```python
from build123d import *

# Parameters (mm, degrees)
SKETCH1_R                = 8.5
BOSS_EXTRUDE1_DEPTH      = 2
BOSS_EXTRUDE2_DEPTH      = 4
BOSS_EXTRUDE2_DEPTH_BACK = 2
CHAMFER1_SIZE            = 1
CHAMFER1_SIZE2           = 2.050303842
CUT_EXTRUDE1_DEPTH       = 1
SKETCH5_W                = 5
SKETCH5_H                = 2.5
BOSS_EXTRUDE3_DEPTH      = 6
CHAMFER2_SIZE            = 3.8


with BuildPart() as part:
    # Sketch1 → Boss-Extrude1 (new body)
    # profile 1 of 2: a face of its own
    with BuildSketch(Plane.XY):
        with BuildLine():
            Line((-22.564385508, -10.000007952), (-6, -10.000007952))
            Line((-6, -10.000007952), (-6, -7.5))
            ThreePointArc((-6, -7.5), (-5.267766953, -5.732233047), (-3.5, -5))
            Line((-3.5, -5), (3.5, -5))
            ThreePointArc((3.5, -5), (5.267766953, -5.732233047), (6, -7.5))
            Line((6, -7.5), (6, -10.000007952))
            Line((6, -10.000007952), (22.435614492, -10.000007952))
            Line((22.435614492, -10.000007952), (22.435614492, 9.999992048))
            Line((22.435614492, 9.999992048), (-22.564385508, 9.999992048))
            Line((-22.564385508, 9.999992048), (-22.564385508, -10.000007952))
        make_face()
        with Locations((-13, 0)):
            Circle(SKETCH1_R, mode=Mode.SUBTRACT)
        with Locations((13, 0)):
            Circle(SKETCH1_R, mode=Mode.SUBTRACT)
    # profile 2 of 2: a face of its own
    with BuildSketch(Plane.XY):
        Polygon((-6, -10.500007952), (-6, -10.000007952), (-22.564385508, -10.000007952), (-22.564385508, 9.999992048), (22.435614492, 9.999992048), (22.435614492, -10.000007952), (6, -10.000007952), (6, -10.500007952), (22.935614492, -10.500007952), (22.935614492, 10.499992048), (-23.064385508, 10.499992048), (-23.064385508, -10.500007952), align=None)
    extrude(amount=BOSS_EXTRUDE1_DEPTH)

    # Sketch2 → Boss-Extrude2 (add, two sides: drawn at the far end of the back side and taken through both)
    with BuildSketch(Plane(origin=(0, 0, 0), x_dir=(-1, 0, 0), z_dir=(0, 0, -1)).offset(-BOSS_EXTRUDE2_DEPTH_BACK)):
        Polygon((6, -12.500007952), (25.064385508, -12.500007952), (25.064385508, 12.499992048), (-24.935614492, 12.499992048), (-24.935614492, -12.500007952), (-6, -12.500007952), (-6, -10.500007952), (-22.935614492, -10.500007952), (-22.935614492, 10.499992048), (23.064385508, 10.499992048), (23.064385508, -10.500007952), (6, -10.500007952), align=None)
    extrude(amount=BOSS_EXTRUDE2_DEPTH + BOSS_EXTRUDE2_DEPTH_BACK)

    # Chamfer1
    chamfer1_edges = [part.edges().sort_by_distance(p)[0] for p in [
        (-15.532192754, -12.500007952, 2),
        (-25.064385508, -7.952e-06, 2),
        (-0.064385508, 12.499992048, 2),
        (24.935614492, -7.952e-06, 2),
        (15.467807246, -12.500007952, 2),
    ]]
    chamfer1_side = [part.faces().sort_by_distance(p)[0] for p in [
        (-0.113559128, 1.090103523, 2),
    ]]
    chamfer(chamfer1_edges, length=CHAMFER1_SIZE, length2=CHAMFER1_SIZE2, reference=chamfer1_side[0])

    # Sketch3 → Cut-Extrude1 (cut)
    with BuildSketch(Plane(origin=(0, 0, 0), x_dir=(-1, 0, 0), z_dir=(0, 0, -1))):
        with BuildLine():
            Line((-5, 9.949992048), (5, 9.949992048))
            ThreePointArc((5, 9.949992048), (6.2, 8.749992048), (5, 7.549992048))
            Line((5, 7.549992048), (-5, 7.549992048))
            ThreePointArc((-5, 7.549992048), (-6.2, 8.749992048), (-5, 9.949992048))
        make_face()
    extrude(amount=-CUT_EXTRUDE1_DEPTH, mode=Mode.SUBTRACT)

    # Sketch5 → Boss-Extrude3 (add)
    with BuildSketch(Plane.XZ.offset(-10.499992048)):
        with Locations((7.5, -5.25)):
            Rectangle(SKETCH5_W, SKETCH5_H)
        Polygon((10, -6.5), (5, -6.5), (5, -9), (12.5, -9), (12.5, -6.5), align=None)
        with Locations((-7.5, -5.25)):
            Rectangle(SKETCH5_W, SKETCH5_H)
        Polygon((-5, -9), (-5, -6.5), (-10, -6.5), (-12.5, -6.5), (-12.5, -9), align=None)
    extrude(amount=-BOSS_EXTRUDE3_DEPTH)

    # Chamfer2
    chamfer2_edges = [part.edges().sort_by_distance(p)[0] for p in [
        (7.5, 12.499992048, -4),
        (-7.5, 12.499992048, -4),
    ]]
    chamfer(chamfer2_edges, length=CHAMFER2_SIZE)


solid = part.part
```
Model file for the job. Use its own axes, mm. A direction names the side the tool comes from. Coordinates: 2 decimals unless noted, no trailing zeros. Loops run counter-clockwise (first coordinate to the right, second up) from the corner with the lowest first, then second, coordinate; pieces in that order, holes last. Notation, with made-up numbers: M 7.5,62 L 14.5,62 A28 cw 14.5,88 Z; hole C 35,15 d6. An arc over 180 degrees is marked long. Use CSV: the item, a comma, the result in double quotes. Start each with the question number.
1. Two-plate mould, pull along Y, no slides. Class faces 1 (the flat face through (-0.1, 7.55, 0.5)), 2 (the flat face through (16, -12.5, -2)), 3 (the flat face through (7.5, 14.4, -2.1)): pulls with the +Y half, pulls with the -Y half, needs draft (parallel to the pull), parting line crosses it, or undercut.
2. Band-saw the part on A-A, the plane z = -7. List the corners of the cut face in (x, y).
3. Tool access for faces 4 (the flat face through (-12.5, 13, -8)), 5 (the flat face through (0.1, 9.95, 0.5)), 6 (the flat face through (12.5, 13, -8)), 7 (the cylindrical face through (-5.287, -5.752, 0.986)): list every direction of +Z, -Z, +X, -X, +Y, -Y with a clear straight run to the whole face (end or side of a thin tool).
4. Band-saw the part on C-C, the plane x = 13. List the corners of the cut face in (y, z).
5. Band-saw the part on B-B, the plane y = -4. List the corners of the cut face in (x, z), then the cut area to 3 significant figures.
6. Probe probe 1 along Y at (x, z) = (-13.5, -3.75); probe 2 along X at (y, z) = (-10.25, -3.5); probe 3 along X at (y, z) = (1, 0.5). List the from-to ranges inside material, lowest first. Write a range as [from, to].
7. Flat gauge pins, fed straight in: pin 1 (0.8 mm diameter, centred on x = 11, y = 14, fed in from +Z); pin 2 (3 mm diameter, centred on y = 14.5, z = -2.5, fed in from +X); pin 3 (1 mm diameter, centred on x = 1.5, y = 12, fed in from -Z). Where does each tip first touch, or does it go through?
8. Band-saw the part on D-D, the plane x = -22. List the corners of the cut face in (y, z), then the cut area to 3 significant figures.
Entries:
1,face 1,"undercut"
1,face 2,"pulls with the -Y half"
1,face 3,"pulls with the +Y half"
2,outline,"M -12.5,10.5 L -5,10.5 L -5,16.5 L -12.5,16.5 Z; M 5,10.5 L 12.5,10.5 L 12.5,16.5 L 5,16.5 Z"
3,face 4,"-Z, -X, +Y, -Y"
3,face 5,"-Z"
3,face 6,"-Z, +X, +Y, -Y"
3,face 7,"+Z, -Z, -Y"
4,outline,"M -12.5,-4 L -10.5,-4 L -10.5,0 L -8.5,0 L -8.5,2 L -11.5,2 L -12.5,-0.05 Z; M 8.5,0 L 10.5,0 L 10.5,-4 L 12.5,-4 L 12.5,-0.05 L 11.5,2 L 8.5,2 Z"
5,outline,"M -25.06,-4 L -23.06,-4 L -23.06,0 L -20.5,0 L -20.5,2 L -24.06,2 L -25.06,-0.05 Z; M -5.5,0 L 5.5,0 L 5.5,2 L -5.5,2 Z; M 20.5,0 L 22.94,0 L 22.94,-4 L 24.94,-4 L 24.94,-0.05 L 23.94,2 L 20.5,2 Z"
5,area,"53.9 mm2"
6,probe 1,"y = [-12.5, -10.5], [10.5, 12.5]"
6,probe 2,"x = [-25.06, -23.06], [22.94, 24.94]"
6,probe 3,"x = [-24.8, -21.44], [-4.56, 4.56], [21.44, 24.67]"
7,pin 1,"stops at z = -6.5"
7,pin 2,"stops at x = 10"
7,pin 3,"stops at z = -4"
8,outline,"M -12.5,-4 L -10.5,-4 L -10.5,0 L 10.5,0 L 10.5,-4 L 12.5,-4 L 12.5,-0.05 L 11.5,2 L -11.5,2 L -12.5,-0.05 Z"
8,area,"63.9 mm2"
